```python
from build123d import *

# Parameters (mm, degrees)
SKETCH1_R                 = 95.25
BOSS_EXTRUDE1_DEPTH       = 23.8125
SKETCH2_R                 = 9.525
BOLTHOLE_DEPTH            = 137.792398021
BOLTHOLEPATTERN_COUNT     = 4
SKETCH5_OUTSIDE_W         = 246.592
SKETCH5_OUTSIDE_H         = 246.592
SKETCH5_OUTSIDE_R         = 63.5
RAISED_FACE_DEPTH         = 1.5875
SKETCH8_R                 = 53.975
WELD_NECK_120_DRAFT_DEPTH = 46.0375
WELD_NECK_120_DRAFT_TAPER = 30
WELD_NECK_END_REACH       = 153.737
SKETCH9_R                 = 44.45
WELD_NECK_CHAMFER1_SIZE   = 2.991731193
WELD_NECK_CHAMFER1_SIZE2  = 3.8989
SKETCH7_R                 = 38.9636
BORE_DEPTH                = 152.737099946
FILLET2_R                 = 1.5875
FILLET3_R                 = 1.5875


with BuildPart() as part:
    # Sketch1 → Boss-Extrude1 (new body)
    with BuildSketch(Plane.XY):
        Circle(SKETCH1_R)
    extrude(amount=BOSS_EXTRUDE1_DEPTH)

    # Sketch2 → BoltHole (cut, through all)
    with BuildSketch(Plane.XY):
        with Locations((53.881536726, 53.881536726)):
            Circle(SKETCH2_R)
    bolthole = extrude(amount=BOLTHOLE_DEPTH, mode=Mode.SUBTRACT)

    # BoltHolePattern: BoltHole ×4 about axis
    boltholepattern_axis = Axis((0, 0, 0), (0, 0, 1))
    for i in range(1, BOLTHOLEPATTERN_COUNT):
        add(bolthole.rotate(boltholepattern_axis, i * 360 / BOLTHOLEPATTERN_COUNT), mode=Mode.SUBTRACT)

    # Sketch5 outside → Raised Face (cut)
    with BuildSketch(Plane(origin=(0, 0, 0), x_dir=(-1, 0, 0), z_dir=(0, 0, -1))):
        Rectangle(SKETCH5_OUTSIDE_W, SKETCH5_OUTSIDE_H)
        Circle(SKETCH5_OUTSIDE_R, mode=Mode.SUBTRACT)
    extrude(amount=-RAISED_FACE_DEPTH, mode=Mode.SUBTRACT)

    # Sketch8 → Weld Neck 120 Draft (add)
    with BuildSketch(Plane.XY.offset(23.8125)):
        Circle(SKETCH8_R)
    extrude(amount=WELD_NECK_120_DRAFT_DEPTH, taper=WELD_NECK_120_DRAFT_TAPER)

    # Sketch9 → Weld Neck End (add, up to next)
    with BuildSketch(Plane.XY.offset(69.85), mode=Mode.PRIVATE) as weld_neck_end_sk1:
        Circle(SKETCH9_R)
    weld_neck_end_tool1 = extrude(weld_neck_end_sk1.sketch, amount=-WELD_NECK_END_REACH, mode=Mode.PRIVATE) - part.part
    add(weld_neck_end_tool1.solids().sort_by_distance((0, 0, 69.85))[0])

    # Weld Neck Chamfer1
    weld_neck_chamfer1_edges = [part.edges().sort_by_distance(p)[0] for p in [
        (-44.45, 0, 69.85),
    ]]
    weld_neck_chamfer1_side = [part.faces().sort_by_distance(p)[0] for p in [
        (-44.45, 0, 55.080141971),
    ]]
    chamfer(weld_neck_chamfer1_edges, length=WELD_NECK_CHAMFER1_SIZE, length2=WELD_NECK_CHAMFER1_SIZE2, reference=weld_neck_chamfer1_side[0])

    # Sketch7 → Bore (cut, through all)
    with BuildSketch(Plane.XY):
        Circle(SKETCH7_R)
    extrude(amount=BORE_DEPTH, mode=Mode.SUBTRACT)

    # Fillet2
    fillet2_edges = [part.edges().sort_by_distance(p)[0] for p in [
        (-95.25, 0, 1.5875),
        (-95.25, 0, 23.8125),
    ]]
    fillet(fillet2_edges, radius=FILLET2_R)

    # Fillet3
    fillet3_edges = [part.edges().sort_by_distance(p)[0] for p in [
        (63.5, 0, 1.5875),
    ]]
    fillet(fillet3_edges, radius=FILLET3_R - 0.0001)  # a hair under: the kernel refuses the full size


solid = part.part
```
Input: part model. Units: mm. Frame: model coordinates. A direction names the side the tool comes from. Coordinates: 2 decimals unless noted, no trailing zeros. Loops run counter-clockwise (first coordinate to the right, second up) from the corner with the lowest first, then second, coordinate; pieces in that order, holes last.
Q1. Section C-C, the plane z = 12. Return the cut outline in (x, y) (3 decimals), and give its area (3 significant figures).
Results are:
outline: circle Ø190.5 at (0, 0); hole circle Ø19.05 at (-53.882, -53.882); hole circle Ø19.05 at (-53.882, 53.882); hole circle Ø77.927 at (0, 0); hole circle Ø19.05 at (53.882, -53.882); hole circle Ø19.05 at (53.882, 53.882)
area: 22,600 mm2
Q2. Contact query for flat-ended pins moving along their axis: pin 1 (3 mm diameter, centred on x = -26.5, y = 31, fed in from -Z); pin 2 (25 mm diameter, centred on x = 53.88, y = -53.88, fed in from -Z); pin 3 (6 mm diameter, centred on x = 41, y = 29.5, fed in from +Z); pin 4 (3 mm diameter, centred on y = 33.5, z = 16.5, fed in from -X). Output: stop coordinate, or through.
Results are:
pin 1: stops at z = 0
pin 2: stops at z = 0.77
pin 3: stops at z = 35.01
pin 4: stops at x = -89.71
Q3. Mould query, pull axis X, two halves, no side actions, for faces 4 (the conical face through (-8.832, -39.772, 69.705)), 5 (the cylindrical face through (-52.642, -63.325, 12.544)), 6 (the flat face through (-21, 33, 69.85)), 7 (the cylindrical face through (63.325, -52.642, 12.544)). Classes: +X half, -X half, draft (parallel to the pull), parting line (faces both ways), or undercut.
Results are:
face 4: parting line
face 5: undercut
face 6: draft
face 7: undercut
Q4. Set-up query: faces 1 (the cylindrical face through (42.397, 13.352, 53.77)), 2 (the flat face through (64, -20, 1.588)), 3 (the cylindrical face through (-75.587, -57.958, 12.567)). Return all of +Z, -Z, +X, -X, +Y, -Y with unobstructed straight access to the full face (end or side cutting, diameter ignored); none if empty.
Results are:
face 1: +Z
face 2: -Z
face 3: +Z, -Z
Q5. Line query: line 1 along Z through (x, y) = (49.5, 64); line 2 along Y through (x, z) = (3, 15.5); line 3 along X through (y, z) = (6, 53). Output: solid intervals per line, ascending.
Results are:
line 1: z = 1.59 to 23.81
line 2: y = -95.2 to -38.85, 38.85 to 95.2
line 3: x = -44.04 to -38.5, 38.5 to 44.04
Q6. Section D-D, the plane x = -59. Give the number of separate pieces and of enclosed holes in the cut face, and give its area (3 significant figures).
Results are:
separate pieces: 3
enclosed holes: 0
area: 2,680 mm2
